Geometry: final body of the model. Coordinates: model frame, mm. Face numbers are marked on the shaded views. A direction names the side the tool comes from. Give positions to 0.01 mm unless a question says otherwise; leave off trailing zeros. Write each loop counter-clockwise with the first axis right and the second up, starting at its lowest first coordinate (ties: lowest second). Pieces come first, ordered by that corner, then holes.
```python
from build123d import *

# Parameters (mm, degrees)
F0_W     = 25
F0_H     = 20
F1_DEPTH = 13
F2_W     = 11.3
F2_H     = 9.8
F3_DEPTH = 11
F4_W     = 20.3
F4_H     = 2.1
F5_DEPTH = 25
F6_R     = 30
F7_DEPTH = 25


with BuildPart() as f1:
    # F0 (on Top) → F1 (new body)
    with BuildSketch(Plane.XY):
        with Locations((-30.473944, -4.285119)):
            Rectangle(F0_W, F0_H)
    extrude(amount=F1_DEPTH)

    # F2 (on face) → F3 (cut)
    with BuildSketch(Plane.XY.offset(13)):
        with Locations((-34.323944, -4.285119)):
            Rectangle(F2_W, F2_H)
    extrude(amount=-F3_DEPTH, mode=Mode.SUBTRACT)

    # F4 (on face) → F5 (cut)
    with BuildSketch(Plane.XY.offset(13)):
        with Locations((-32.823944, 4.664881)):
            Rectangle(F4_W, F4_H)
        with Locations((-32.823944, -13.235119)):
            Rectangle(F4_W, F4_H)
    extrude(amount=-F5_DEPTH, mode=Mode.SUBTRACT)

    # F6 (on face) → F7 (cut)
    with BuildSketch(Plane.XY.offset(13)):
        with Locations((10.326056, -4.285119)):
            Circle(F6_R)
    extrude(amount=-F7_DEPTH, mode=Mode.SUBTRACT)


solid = f1.part
```
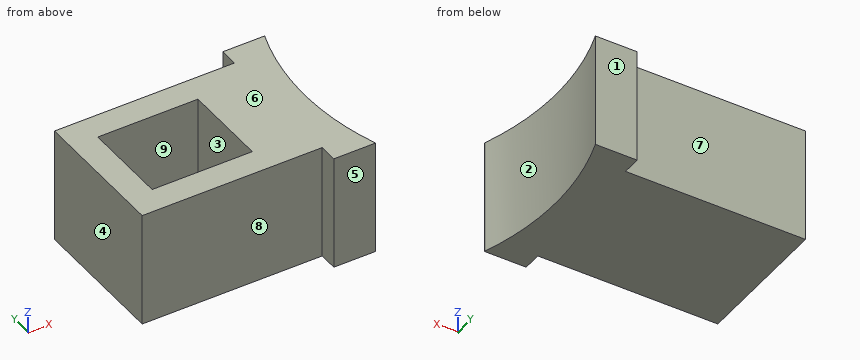
Item 1: Section B-B, the plane x = -34.5. Return the cut outline in (y, z), plus the area to 3 significant figures.
Found:
outline: (-12.19, 0) - (3.61, 0) - (3.61, 13) - (0.61, 13) - (0.61, 2) - (-9.19, 2) - (-9.19, 13) - (-12.19, 13) - close
area: 97.6 mm2
Item 2: Reachability of the marked faces 5, 6, 7, 8 and 9 from +Z, -Z, +X, -X, +Y, -Y: full face, straight path, thin tool, end or side. Return the list, or none.
Found:
face 5: +Z, -Z, +X, -X, -Y
face 6: +Z, +X, -X, +Y, -Y
face 7: +Z, -Z, -X, +Y
face 8: +Z, -Z, -X, -Y
face 9: +Z
Item 3: Pin query (flat end, axial travel): pin 1 Ø4 at (x, z) = (-31, 9.5) entering from -Y; pin 2 Ø3 at (x, y) = (-32.5, -4.5) entering from +Z; pin 3 Ø0.6 at (y, z) = (4.5, 6) entering from -X. Return the tip coordinate at first contact, or that it passes through.
Found:
pin 1: stops at y = -12.19
pin 2: stops at z = 2
pin 3: stops at x = -22.67
Item 4: Line query: L1, parallel to Y at x = -28.75, z = 8.25; L2, parallel to Z at x = -37.25, y = -7.75; L3, parallel to Y at x = -28.5, z = 11. Output: solid intervals per line, ascending.
Found:
L1: y = -12.19 to -9.19, 0.61 to 3.61
L2: z = 0 to 2
L3: y = -12.19 to 3.61
Item 5: Section A-A, the plane z = 5. Return the cut outline in (x, y), plus the area to 3 significant figures.
Found:
outline: (-42.97, -12.19) - (-22.67, -12.19) - (-22.67, -14.29) - (-17.97, -14.29) - (-17.97, -14.24) arc R30 cw to (-17.97, 5.67) - (-17.97, 5.71) - (-22.67, 5.71) - (-22.67, 3.61) - (-42.97, 3.61) - close; hole (-39.97, -9.19) - (-28.67, -9.19) - (-28.67, 0.61) - (-39.97, 0.61) - close
area: 281 mm2
Item 6: Section D-D, the plane x = -28.25. Return the cut outline in (y, z), plus the area to 3 significant figures.
Found:
outline: (-12.19, 0) - (3.61, 0) - (3.61, 13) - (-12.19, 13) - close
area: 205 mm2
Item 7: Section C-C, the plane y = -8.25. Return the cut outline in (x, z), plus the area to 3 significant figures.
Found:
outline: (-42.97, 0) - (-19.41, 0) - (-19.41, 13) - (-28.67, 13) - (-28.67, 2) - (-39.97, 2) - (-39.97, 13) - (-42.97, 13) - close
area: 182 mm2
Item 8: Pull-direction query (X, two-part tool) for the marked faces 1, 2, 3 and 4; classes: +X half, -X half, draft (parallel to the pull), parting line (faces both ways), or undercut.
Found:
face 1: draft
face 2: +X half
face 3: undercut
face 4: -X half
